Read the model definition and answer for the solid it produces. Units are mm, in the model's axes. Face numbers are marked on the shaded views. Coordinates: 2 decimals unless noted, no trailing zeros. Write each loop counter-clockwise with the first axis right and the second up, starting at its lowest first coordinate (ties: lowest second). Pieces come first, ordered by that corner, then holes. Notation, with made-up numbers: (10, 54) - (49, 54) arc R20 ccw to (49, 82) - close; hole circle Ø6 at (-17.5, 68). An arc over 180 degrees is marked (long way). Return JSON: item names as keys, results as strings.
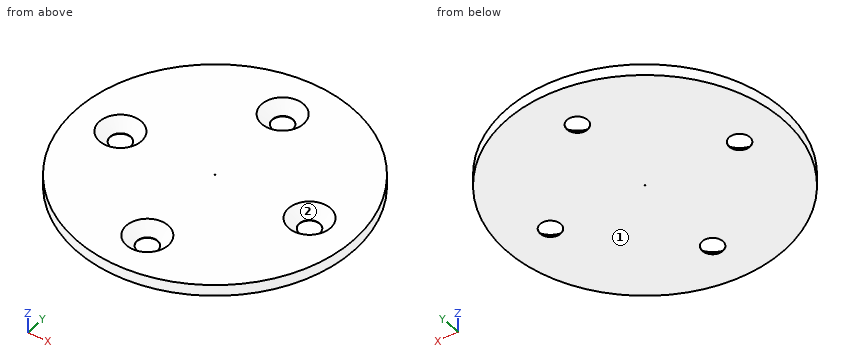
```python
from build123d import *

# Parameters (mm, degrees)
F0_R           = 37
F1_DEPTH       = 3
F3_D           = 5.5
F3_DEPTH       = 15
F3_CSINK_D     = 11.2
F3_CSINK_ANGLE = 90
F3_TIP         = 1.6523667023
F5_D           = 0.2


with BuildPart() as f1:
    # F0 (on Top) → F1 (new body)
    with BuildSketch(Plane.XY):
        Circle(F0_R)
    extrude(amount=F1_DEPTH)

    # F3
    with Locations(Plane.XY.offset(3)):
        with Locations((0, 25), (-25, 0), (0, -25), (25, 0)):
            CounterSinkHole(F3_D / 2, F3_CSINK_D / 2, depth=F3_DEPTH, counter_sink_angle=F3_CSINK_ANGLE)
            with Locations((0, 0, -(F3_DEPTH + F3_TIP / 2))):  # 118° drill point
                Cone(0, F3_D / 2, F3_TIP, mode=Mode.SUBTRACT)

    # F5 (through all)
    with Locations(Plane.XY.offset(3)):
        with Locations((0, 0)):
            Hole(F5_D / 2)


solid = f1.part
```
(1) Determine the mould class of the marked faces 1 and 2 for opening direction X: +X half, -X half, draft (parallel to the pull), parting line (faces both ways), or undercut.
Answer:
{"face 1": "draft", "face 2": "undercut"}
(2) Straight lines are drawn through the part: line 1 (Y direction, x = 25, z = 0.1); line 2 (Y direction, x = -22.5, z = 0.95). For each, find the intervals that lie inside material, in ascending order. Write a range as from..to.
Answer:
{"line 1": "-27.28..-2.75, 2.75..27.28", "line 2": "-29.37..-2.52, 2.52..29.37"}
(3) A cutting plane is placed at D-D (x = -1). State how many separate pieces and enclosed holes the cut face has, and give its area (3 significant figures).
Answer:
{"separate pieces": "3", "enclosed holes": "0", "area": "174 mm²"}
(4) A cutting plane is placed at C-C (y = -9). Determine the outline of the cut face in (x, z).
Answer:
{"outline": "(-35.89, 0) - (35.89, 0) - (35.89, 3) - (-35.89, 3) - close"}
(5) Flat-ended cylindrical pins translate along their axes: P1, Ø1, axis at x = -16.5, z = 1, coming from the +Y side; P2, Ø9, axis at x = -25, y = 0, coming from the +Z side. Find the tip coordinate at first contact, or state that the pin passes through.
Answer:
{"P1": "y = 33.36", "P2": "z = 1.9"}
(6) A cutting plane is placed at B-B (x = 25). Determine the outline of the cut face in (y, z).
Answer:
{"outline": "(-27.28, 0) - (-2.75, 0) - (-2.75, 0.15) - (-5.6, 3) - (-27.28, 3) - close; (2.75, 0) - (27.28, 0) - (27.28, 3) - (5.6, 3) - (2.75, 0.15) - close"}
(7) A cutting plane is placed at A-A (z = 2.45). Determine the outline of the cut face in (x, y), and give its area (3 significant figures).
Answer:
{"outline": "circle Ø74 at (0, 0); hole circle Ø10.1 at (-25, 0); hole circle Ø10.1 at (0, -25); hole circle Ø10.1 at (0, 25); hole circle Ø0.2 at (0, 0); hole circle Ø10.1 at (25, 0)", "area": "3,980 mm²"}
